```python
from build123d import *

# Parameters (mm, degrees)
SKETCH1_W                      = 25.4
SKETCH1_H                      = 15.875
BOSS_EXTRUDE1_DEPTH            = 459.74
SKETCH8_R                      = 6.8199
CUT_EXTRUDE1_DEPTH             = 22.61362
L_0_29_DIAMETER_HOLE1_D        = 7.366
L_0_29_DIAMETER_HOLE1_DEPTH    = 50.8
L_0_29_DIAMETER_HOLE1_TIP      = 2.21296966
TAP_DRILL_FOR_10_24_TAP2_D     = 3.7973
TAP_DRILL_FOR_10_24_TAP2_DEPTH = 20.701
TAP_DRILL_FOR_10_24_TAP2_TIP   = 1.140824014
TAP_DRILL_FOR_10_24_TAP1_D     = 3.7973
TAP_DRILL_FOR_10_24_TAP1_DEPTH = 20.701
TAP_DRILL_FOR_10_24_TAP1_TIP   = 1.140824014


with BuildPart() as part:
    # Sketch1 → Boss-Extrude1 (new body)
    with BuildSketch(Plane.XY):
        with Locations((12.7, 7.9375)):
            Rectangle(SKETCH1_W, SKETCH1_H)
    extrude(amount=BOSS_EXTRUDE1_DEPTH)

    # Sketch8 → Cut-Extrude1 (cut)
    with BuildSketch(Plane.ZY):
        with Locations((434.34, 7.9375)):
            Circle(SKETCH8_R)
        with Locations((25.4, 7.9375)):
            Circle(SKETCH8_R)
    extrude(amount=-CUT_EXTRUDE1_DEPTH, mode=Mode.SUBTRACT)

    # L (0.29) Diameter Hole1
    with Locations(Plane.ZY.offset(-22.61362)):
        with Locations((25.4, 7.9375), (434.34, 7.9375)):
            Hole(L_0_29_DIAMETER_HOLE1_D / 2, depth=L_0_29_DIAMETER_HOLE1_DEPTH)
            with Locations((0, 0, -(L_0_29_DIAMETER_HOLE1_DEPTH + L_0_29_DIAMETER_HOLE1_TIP / 2))):  # 118° drill point
                Cone(0, L_0_29_DIAMETER_HOLE1_D / 2, L_0_29_DIAMETER_HOLE1_TIP, mode=Mode.SUBTRACT)

    # Tap Drill for #10-24 Tap2
    with Locations(Plane(origin=(-2202.638131805, 879.599136144, 459.74), x_dir=(0, 1, 0), z_dir=(0, 0, 1))):
        with Locations((-871.661636144, -2222.038131805), (-871.661636144, -2208.638131805)):
            Hole(TAP_DRILL_FOR_10_24_TAP2_D / 2, depth=TAP_DRILL_FOR_10_24_TAP2_DEPTH)
            with Locations((0, 0, -(TAP_DRILL_FOR_10_24_TAP2_DEPTH + TAP_DRILL_FOR_10_24_TAP2_TIP / 2))):  # 118° drill point
                Cone(0, TAP_DRILL_FOR_10_24_TAP2_D / 2, TAP_DRILL_FOR_10_24_TAP2_TIP, mode=Mode.SUBTRACT)

    # Tap Drill for #10-24 Tap1
    with Locations(Plane(origin=(0, 0, 0), x_dir=(-1, 0, 0), z_dir=(0, 0, -1))):
        with Locations((-19.4, 7.9375), (-6, 7.9375)):
            Hole(TAP_DRILL_FOR_10_24_TAP1_D / 2, depth=TAP_DRILL_FOR_10_24_TAP1_DEPTH)
            with Locations((0, 0, -(TAP_DRILL_FOR_10_24_TAP1_DEPTH + TAP_DRILL_FOR_10_24_TAP1_TIP / 2))):  # 118° drill point
                Cone(0, TAP_DRILL_FOR_10_24_TAP1_D / 2, TAP_DRILL_FOR_10_24_TAP1_TIP, mode=Mode.SUBTRACT)


solid = part.part
```
Read the model definition and answer for the solid it produces. Units are mm, in the model's axes. A direction names the side the tool comes from. Coordinates: 2 decimals unless noted, no trailing zeros. Write each loop counter-clockwise with the first axis right and the second up, starting at its lowest first coordinate (ties: lowest second). Pieces come first, ordered by that corner, then holes. Notation, with made-up numbers: (-33.5, 67) -> (24.5, 67) arc R16 ccw to (24.5, 92) -> close; hole circle Ø7 at (73, 61). An arc over 180 degrees is marked (long way). Return JSON: item names as keys, results as strings.
1. Each of these flat-tipped pins is pushed along its axis until it touches: P1, Ø12, axis at x = 15, z = 126.5, coming from the -Y side; P2, Ø8.5, axis at y = 7.94, z = 25.4, coming from the -X side; P3, Ø4, axis at y = 8.5, z = 433.5, coming from the -X side; P4, Ø3, axis at x = 19.4, y = 7.94, coming from the +Z side. Where does it stop, or does it pass through?
Found:
{"P1": "y = 0", "P2": "x = 22.61", "P3": "through", "P4": "z = 427.69"}
2. Find the intervals of material crossed by line 1 along Z through (x, y) = (1.25, 8.5); line 2 along Z through (x, y) = (12.25, 8.75); line 3 along Y through (x, z) = (7.25, 25.4) (3 decimals), in increasing order. Write a range as from..to.
Found:
{"line 1": "0..18.6, 32.2..427.54, 441.14..459.74", "line 2": "0..18.63, 32.17..427.57, 441.11..459.74", "line 3": "0..1.118, 14.757..15.875"}
3. A cutting plane is placed at A-A (x = 13.5). Determine the outline of the cut face in (y, z) (1 decimal).
Found:
{"outline": "(0, 0) -> (15.9, 0) -> (15.9, 459.7) -> (0, 459.7) -> close; hole circle Ø13.6 at (7.9, 25.4); hole circle Ø13.6 at (7.9, 434.3)"}
4. A tool of negligible diameter and unlimited length cuts with its end or side. For faces 4 (the face through (13, 8, 459.74)), 5 (the face through (11.149, 8.237, 427.527)), from which of +Z, -Z, +X, -X, +Y, -Y can it reach the whole face along a straight path? Write none if from no direction.
Found:
{"face 4": "+Z, +X, -X, +Y, -Y", "face 5": "-X"}
5. Determine the mould class of faces 1 (the face through (13, 8, 0)), 2 (the face through (24.026, 5.696, 437.263)), 3 (the face through (13, 0, 227)) for opening direction Y: pulls with the +Y half, pulls with the -Y half, needs draft (parallel to the pull), parting line crosses it, or undercut.
Found:
{"face 1": "needs draft", "face 2": "undercut", "face 3": "pulls with the -Y half"}
